```python
from build123d import *

# Parameters (mm, degrees)
SZKIC1_W                    = 5
SZKIC1_H                    = 10
DODANIE_WYCI_GNI_CIE1_DEPTH = 1
DODANIE_WYCI_GNI_CIE4_DEPTH = 4
ZAOKR_GLENIE2_R             = 5
SZKIC3_W                    = 1
SZKIC3_H                    = 4
WYTNIJ_WYCI_GNI_CIE1_DEPTH  = 4
SZKIC4_W                    = 0.5
SZKIC4_H                    = 4
DODANIE_WYCI_GNI_CIE5_DEPTH = 1
SZKIC5_R                    = 0.25
DODANIE_WYCI_GNI_CIE6_DEPTH = 2
SZKIC6_R                    = 0.55
SZKIC6_R_2                  = 0.5
DODANIE_WYCI_GNI_CIE7_DEPTH = 0.5
SZKIC7_W                    = 7
SZKIC7_H                    = 1
DODANIE_WYCI_GNI_CIE8_DEPTH = 1
SZKIC11_R                   = 0.25
WYTNIJ_WYCI_GNI_CIE2_DEPTH  = 0.5
SZKIC14_R                   = 0.125
WYTNIJ_WYCI_GNI_CIE3_DEPTH  = 1


with BuildPart() as part:
    # Szkic1 → Dodanie-wyciągnięcie1 (new body)
    with BuildSketch(Plane(origin=(0, 0, 0), x_dir=(1, 0, 0), z_dir=(0, 1, 0))):
        Rectangle(SZKIC1_W, SZKIC1_H)
    extrude(amount=DODANIE_WYCI_GNI_CIE1_DEPTH)

    # Szkic2 → Dodanie-wyciągnięcie4 (add)
    with BuildSketch(Plane(origin=(0, 1, 0), x_dir=(1, 0, 0), z_dir=(0, 1, 0))):
        Polygon((-2.5, 5), (2.5, 5), (2.5, 3.5), (-0.5, 3.5), (-0.5, -3.5), (2.5, -3.5), (2.5, -5), (-2.5, -5), align=None)
    extrude(amount=DODANIE_WYCI_GNI_CIE4_DEPTH)

    # Zaokrąglenie2
    zaokr_glenie2_edges = [part.edges().sort_by_distance(p)[0] for p in [
        (-2.5, 2.5, -5),
        (-2.5, 2.5, 5),
    ]]
    fillet(zaokr_glenie2_edges, radius=ZAOKR_GLENIE2_R - 0.0001)  # a hair under: the kernel refuses the full size

    # Szkic3 → Wytnij-wyciągnięcie1 (cut)
    with BuildSketch(Plane(origin=(0, 1, 0), x_dir=(1, 0, 0), z_dir=(0, 1, 0))):
        with Locations((0.5, 0)):
            Rectangle(SZKIC3_W, SZKIC3_H)
    extrude(amount=-WYTNIJ_WYCI_GNI_CIE1_DEPTH, mode=Mode.SUBTRACT)

    # Szkic4 → Dodanie-wyciągnięcie5 (add)
    with BuildSketch(Plane(origin=(0, 1, 0), x_dir=(1, 0, 0), z_dir=(0, 1, 0))):
        with Locations((-0.25, 0)):
            Rectangle(SZKIC4_W, SZKIC4_H)
    extrude(amount=DODANIE_WYCI_GNI_CIE5_DEPTH)

    # Szkic5 → Dodanie-wyciągnięcie6 (add)
    with BuildSketch(Plane(origin=(0, 1, 0), x_dir=(1, 0, 0), z_dir=(0, 1, 0))):
        with Locations(Location((1.75, 0, 0), (0, 0, 90))):
            Circle(SZKIC5_R)
    extrude(amount=DODANIE_WYCI_GNI_CIE6_DEPTH)

    # Szkic6 → Dodanie-wyciągnięcie7 (add)
    with BuildSketch(Plane(origin=(0, 1, 0), x_dir=(1, 0, 0), z_dir=(0, 1, 0))):
        with Locations(Location((1.75, 0, 0), (0, 0, 90))):
            Circle(SZKIC6_R)
        with Locations(Location((1.75, 0, 0), (0, 0, 270))):
            Circle(SZKIC6_R_2, mode=Mode.SUBTRACT)
    extrude(amount=DODANIE_WYCI_GNI_CIE7_DEPTH)

    # Szkic7 → Dodanie-wyciągnięcie8 (add)
    with BuildSketch(Plane(origin=(-0.5, 0, 0), x_dir=(0, 0, -1), z_dir=(1, 0, 0))):
        with Locations((0, 4.5)):
            Rectangle(SZKIC7_W, SZKIC7_H)
    extrude(amount=DODANIE_WYCI_GNI_CIE8_DEPTH)

    # Szkic11 → Wytnij-wyciągnięcie2 (cut)
    with BuildSketch(Plane(origin=(2.5, 0, 0), x_dir=(0, 0, -1), z_dir=(1, 0, 0))):
        with Locations((4.25, 3.503110499)):
            Circle(SZKIC11_R)
        with Locations((4.25, 1.503110499)):
            Circle(SZKIC11_R)
        with Locations((-4.25, 3.503110499)):
            Circle(SZKIC11_R)
        with Locations((-4.25, 1.503110499)):
            Circle(SZKIC11_R)
    extrude(amount=-WYTNIJ_WYCI_GNI_CIE2_DEPTH, mode=Mode.SUBTRACT)

    # Szkic14 → Wytnij-wyciągnięcie3 (cut)
    with BuildSketch(Plane(origin=(0, 0, 0), x_dir=(0, 0, -1), z_dir=(1, 0, 0))):
        with Locations((0, 1.5)):
            Circle(SZKIC14_R)
    extrude(amount=-WYTNIJ_WYCI_GNI_CIE3_DEPTH, mode=Mode.SUBTRACT)


solid = part.part
```
Build history of the part. All positions in model axes, mm. A direction names the side the tool comes from. Round coordinates to 2 decimals unless told otherwise and drop trailing zeros. Write each loop counter-clockwise with the first axis right and the second up, starting at its lowest first coordinate (ties: lowest second). Pieces come first, ordered by that corner, then holes. Notation, with made-up numbers: (-24.75, 49.5) - (-15.75, 49.5) arc R33 cw to (-15.75, 85.5) - close; hole circle Ø10 at (42, 21.25). An arc over 180 degrees is marked (long way). Answer as CSV lines item,"result".
Q1. Drop flat-ended pins along their axis: pin 1 (0.8 mm diameter, centred on x = 0, z = 0.5, fed in from -Y); pin 2 (0.5 mm diameter, centred on x = 1.5, z = 0, fed in from +Y); pin 3 (0.6 mm diameter, centred on x = 0, y = 1.5, fed in from -Z); pin 4 (0.9 mm diameter, centred on y = 2.5, z = -1, fed in from +X). Give the stop position or say it passes through.
Report:
pin 1,"stops at y = 0"
pin 2,"stops at y = 3"
pin 3,"stops at z = -4.49"
pin 4,"stops at x = -0.5"
Q2. Cut at C-C (z = -1.5). Write the cut outline in (x, y).
Report:
outline,"(-2.27, 0) - (0, 0) - (0, 2) - (-0.5, 2) - (-0.5, 4) - (0.5, 4) - (0.5, 5) - (-2.27, 5) - close; (1, 0) - (2.5, 0) - (2.5, 1) - (1, 1) - close"
Q3. Tool access for faces 4 (the flat face through (-1, 5, 0)), 5 (the flat face through (0.5, 0.5, -2)), 6 (the cylindrical face through (-1.07, 2.54, 3.5)), 7 (the flat face through (0.5, 4.5, 0)), 8 (the flat face through (0, 4, 0)): list every direction of +Z, -Z, +X, -X, +Y, -Y with a clear straight run to the whole face (end or side of a thin tool).
Report:
face 4,"+Z, -Z, +X, -X, +Y"
face 5,"-Y"
face 6,"+Z, -X, +Y, -Y"
face 7,"+X, +Y"
face 8,"+X"
Q4. Pull direction Z, two halves, no side cores. Call faces 1 (the cylindrical face through (-1, 2.54, -3.57)), 2 (the flat face through (2.5, 0.8, -0.1)), 3 (the flat face through (0, 1, 0)): +Z half, -Z half, draft (parallel to the pull), parting line (faces both ways), or undercut.
Report:
face 1,"-Z half"
face 2,"draft"
face 3,"undercut"
Q5. Cut at D-D (x = 1.75). Write the cut outline in (y, z).
Report:
outline,"(0, -4.94) - (5, -4.94) - (5, -3.5) - (1, -3.5) - (1, -0.55) - (1.5, -0.55) - (1.5, -0.5) - (1, -0.5) - (1, -0.25) - (3, -0.25) - (3, 0.25) - (1, 0.25) - (1, 0.5) - (1.5, 0.5) - (1.5, 0.55) - (1, 0.55) - (1, 3.5) - (5, 3.5) - (5, 4.94) - (0, 4.94) - close"
Q6. Drill centre lines: probe 1 along Y at (x, z) = (2.1, -4.25); probe 2 along X at (y, z) = (0.55, 0); probe 3 along Y at (x, z) = (1, -2.25). Where is each one in solid material? Low to high. Write a range as [from, to].
Report:
probe 1,"y = [0, 1.25], [1.75, 3.25], [3.75, 5]"
probe 2,"x = [-2.5, 0], [1, 2.5]"
probe 3,"y = [0, 1]"
